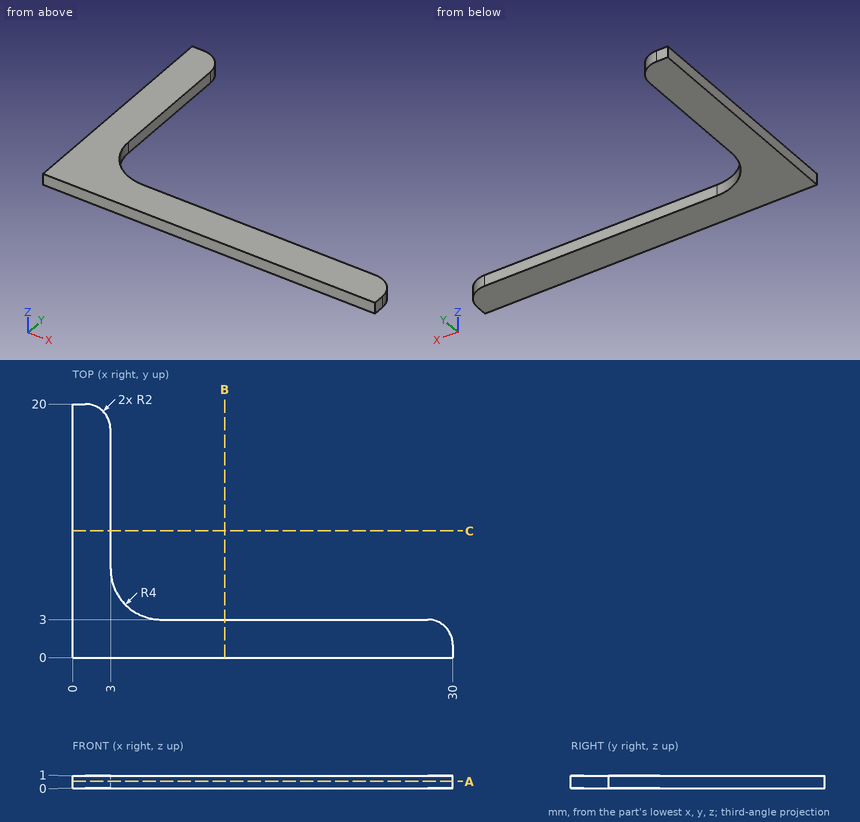
Geometry check sheet. Reference: drawing and pictorial views, mm from the part's lowest x, y, z. Coordinates: 2 decimals unless noted, no trailing zeros. Order: outer loops, then holes, each group sorted by start corner. A loop starts at its lowest first (then second) coordinate and runs counter-clockwise, first axis right, second up.
Item 1: Section check B-B (x = 12). Enter the section's corners in (y, z).
Item 2: Section check A-A (z = 0.55). Enter the section's corners in (x, y), plus the area to 3 significant figures.
Item 3: Depth check by flat-ended pin: pin 1 (2 mm diameter, centred on x = 5.5, y = 9.5, fed in from +Z). Enter the tip coordinate at first touch or a pass-through.
Item 4: Scan lines: line 1 along Y through (x, z) = (12.75, 0.95); line 2 along X through (y, z) = (5.5, 0.9). Record each from-to range of solid material in increasing order.
Check sheet entries:
1. outline: (0, 0) - (3, 0) - (3, 1) - (0, 1) - close
2. outline: (0, 0) - (30, 0) - (30, 1) arc R2 ccw to (28, 3) - (7, 3) arc R4 cw to (3, 7) - (3, 18) arc R2 ccw to (1, 20) - (0, 20) - close
2. area: 143 mm2
3. pin 1: passes through
4. line 1: y = 0 to 3
4. line 2: x = 0 to 3.29
